Design review of the part built by this model. Coordinates are the model's own, in mm. Coordinates: 2 decimals unless noted, no trailing zeros. Write each loop counter-clockwise with the first axis right and the second up, starting at its lowest first coordinate (ties: lowest second). Pieces come first, ordered by that corner, then holes.
Q1. Take a section at B-B (z = -178). Give the boundary of the cut face in (x, y) (3 decimals), and give its area (3 significant figures).
Q2. Take a section at A-A (x = 3.25). Give the boundary of the cut face in (y, z) (3 decimals), and give its area (3 significant figures).
Q3. For probe 1 along Y at (x, z) = (-6.5, -176) (3 decimals), list the stretches that pass through material, from the lowest coordinate up.
Autodesk Inventor part; units mm, degrees
ref_plane "YZ Plane" through (0, 0, 0) normal (1, 0, 0) x (0, 1, 0)
ref_plane "XZ Plane" through (0, 0, 0) normal (0, 1, 0) x (-1, 0, 0)
ref_plane "XY Plane" through (0, 0, 0) normal (0, 0, 1) x (1, 0, 0)
sketch "Sketch2" plane through (0, 0, 0) normal (0, 0, 1) x (1, 0, 0)
  line L0 (-12.7, -12.7) -> (12.7, -12.7)
  line L1 (12.7, -12.7) -> (12.7, 12.7)
  line L2 (12.7, 12.7) -> (-12.7, 12.7)
  line L3 (-12.7, 12.7) -> (-12.7, -12.7)
  line L4 (-12.7, -12.7) -> (12.7, 12.7) construction
  line L5 (12.7, -12.7) -> (-12.7, 12.7) construction
  line L6 (-9.525, -9.525) -> (9.525, -9.525)
  line L7 (9.525, -9.525) -> (9.525, 9.525)
  line L8 (9.525, 9.525) -> (-9.525, 9.525)
  line L9 (-9.525, 9.525) -> (-9.525, -9.525)
  line L10 (-9.525, -9.525) -> (9.525, 9.525) construction
  line L11 (9.525, -9.525) -> (-9.525, 9.525) construction
  point P0 (0, 0)
  dimension "d0" = 25.4
  dimension "d1" = 25.4
  dimension "d2" = 3.175
  dimension "d3" = 3.175
extrude "Extrusion1" add sketch "Sketch2" along normal mid plane 879.856
properties part number "aluminumExtrusion" material "Aluminum 6061-AHC"
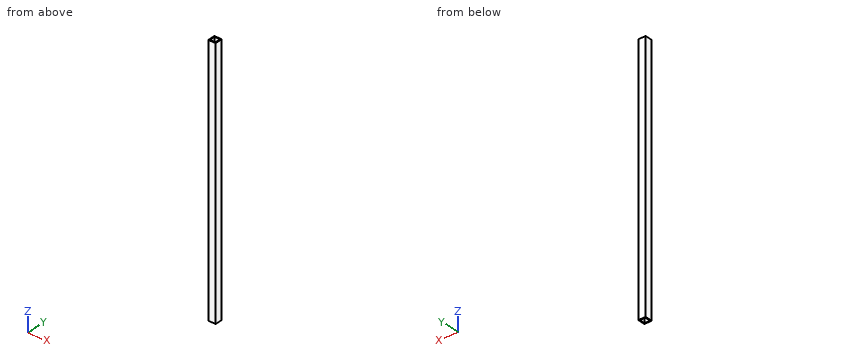
Response:
1. outline: (-12.7, -12.7) - (12.7, -12.7) - (12.7, 12.7) - (-12.7, 12.7) - close; hole (-9.525, -9.525) - (9.525, -9.525) - (9.525, 9.525) - (-9.525, 9.525) - close
1. area: 282 mm2
2. outline: (-12.7, -439.928) - (-9.525, -439.928) - (-9.525, 439.928) - (-12.7, 439.928) - close; (9.525, -439.928) - (12.7, -439.928) - (12.7, 439.928) - (9.525, 439.928) - close
2. area: 5,590 mm2
3. probe 1: y = -12.7 to -9.525, 9.525 to 12.7
